Geometry: final body of the model. Coordinates: model frame, mm. Coordinates: 2 decimals unless noted, no trailing zeros. Loops run counter-clockwise (first coordinate to the right, second up) from the corner with the lowest first, then second, coordinate; pieces in that order, holes last. Notation, with made-up numbers: M 48.5,2.5 L 107.5,2.5 A22 ccw 107.5,10.5 Z; hole C 37,58 d10. An arc over 180 degrees is marked long. Write item = value, one per line. Start each with the question number.
```python
from build123d import *

# Parameters (mm, degrees)
SKETCH1_R           = 1
BOSS_EXTRUDE1_DEPTH = 2


with BuildPart() as part:
    # Sketch1 → Boss-Extrude1 (new body)
    with BuildSketch(Plane.XY):
        with BuildLine():
            Line((0, 0), (9.846049894, 29.538149682))
            ThreePointArc((9.846049894, 29.538149682), (9.961262373, 30.006286251), (10, 30.486832981))
            Line((10, 30.486832981), (10, 107))
            ThreePointArc((10, 107), (9.121320344, 109.121320344), (7, 110))
            Line((7, 110), (-7, 110))
            ThreePointArc((-7, 110), (-9.121320344, 109.121320344), (-10, 107))
            Line((-10, 107), (-10, 30.486832981))
            ThreePointArc((-10, 30.486832981), (-9.961262373, 30.006286251), (-9.846049894, 29.538149682))
            Line((-9.846049894, 29.538149682), (0, 0))
        make_face()
        with Locations((0, 100)):
            Circle(SKETCH1_R, mode=Mode.SUBTRACT)
    extrude(amount=BOSS_EXTRUDE1_DEPTH)


solid = part.part
```
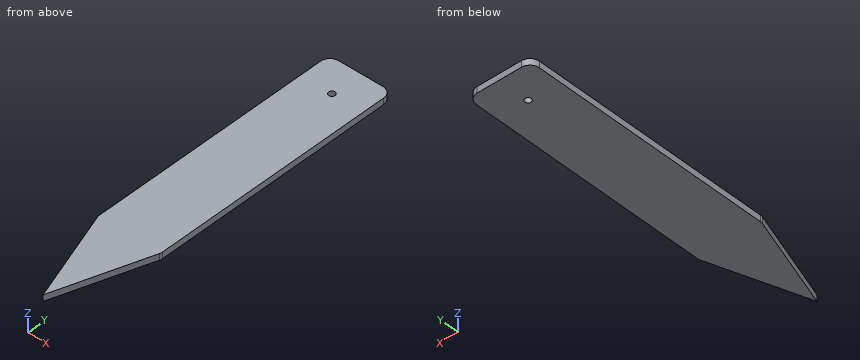
Item 1: Section query C-C (x = -5). Return the cut outline in (y, z), plus the area to 3 significant figures.
Item 2: First-contact query: pin 1 (5 mm diameter, centred on x = -3.5, y = 38, fed in from -Z). Flat tip, straight axial feed; report the tip coordinate or a pass-through.
Item 3: Line query: line 1 (X direction, y = 100, z = 1.45); line 2 (X direction, y = 14.5, z = 1.9); line 3 (X direction, y = 13, z = 1.95). Output: solid intervals per line, ascending. Write a range as from..to.
Item 4: Section query D-D (y = 15). Return the cut outline in (x, z), plus the area to 3 significant figures.
Item 5: Section query B-B (z = 1.3). Return the cut outline in (x, y), plus the area to 3 significant figures.
Item 6: Section query A-A (y = 100). Return the cut outline in (x, z), plus the area to 3 significant figures.
Verdict:
q1.outline = M 15,0 L 110,0 L 110,2 L 15,2 Z
q1.area = 190 mm2
q2.pin_1 = 0
q3.line_1 = -10..-1, 1..10
q3.line_2 = -4.83..4.83
q3.line_3 = -4.33..4.33
q4.outline = M -5,0 L 5,0 L 5,2 L -5,2 Z
q4.area = 20.0 mm2
q5.outline = M -10,30.49 A3 ccw -9.85,29.54 L 0,0 L 9.85,29.54 A3 ccw 10,30.49 L 10,107 A3 ccw 7,110 L -7,110 A3 ccw -10,107 Z; hole C 0,100 d2
q5.area = 1,890 mm2
q6.outline = M -10,0 L -1,0 L -1,2 L -10,2 Z; M 1,0 L 10,0 L 10,2 L 1,2 Z
q6.area = 36.0 mm2
